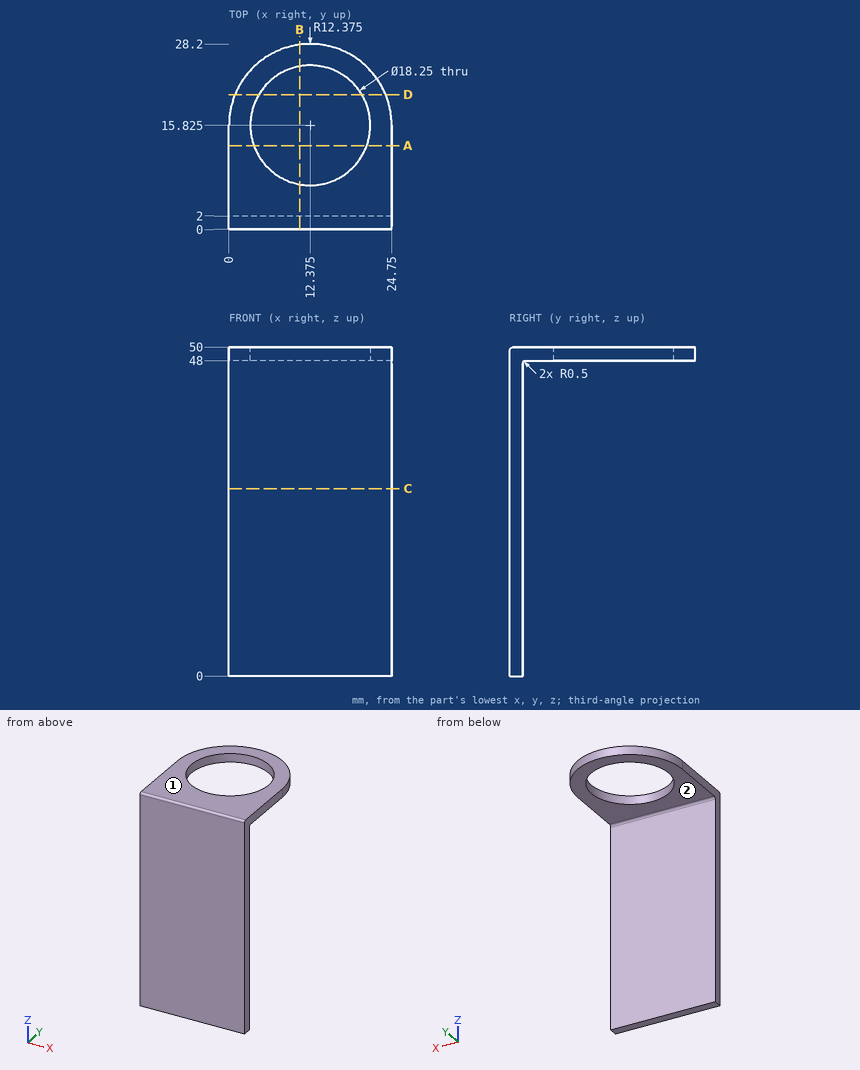
Input: dimensioned drawing with shaded views. Units: mm. Origin: part minimum x, y, z. A direction names the side the tool comes from. Round coordinates to 2 decimals unless told otherwise and drop trailing zeros. Loops run counter-clockwise (first coordinate to the right, second up) from the corner with the lowest first, then second, coordinate; pieces in that order, holes last. Notation, with made-up numbers: (36, -21.5) -> (88, -21.5) arc R17 cw to (88, -15.5) -> close; hole circle Ø3 at (-16, 8). An arc over 180 degrees is marked (long way). Answer as a JSON object with one key per item and string values. Group by question number.
1) Section query C-C on z = 28.5. Output: boundary loops of the cut face in (x, y).
2) Pin query (flat end, axial travel): pin 1 (10 mm diameter, centred on x = 21.5, z = 17.5, fed in from +Y); pin 2 (1.5 mm diameter, centred on x = 21.5, y = 8.5, fed in from -Z); pin 3 (1.5 mm diameter, centred on x = 5.5, y = 15.5, fed in from -Z) (1 decimal). Return the tip coordinate at first contact, or that it passes through.
3) Section query D-D on y = 20.5. Output: boundary loops of the cut face in (x, z), plus the area to 3 significant figures.
4) Ray query, L1, parallel to Z at x = 6, y = 4.5; L2, parallel to Y at x = 6, z = 44. Return the intervals inside material, ascending.
5) Reachability of the marked faces 1 and 2 from +Z, -Z, +X, -X, +Y, -Y: full face, straight path, thin tool, end or side. Return the list, or none.
6) Section query A-A on y = 12.75. Output: boundary loops of the cut face in (x, z), plus the area to 3 significant figures.
7) Section query B-B on x = 10.75. Output: boundary loops of the cut face in (y, z).
Reply:
{
 "1": {"outline": "(0, 0) -> (24.75, 0) -> (24.75, 2) -> (0, 2) -> close"},
 "2": {"pin 1": "stops at y = 2", "pin 2": "stops at z = 48", "pin 3": "passes through"},
 "3": {"outline": "(0.92, 48) -> (4.54, 48) -> (4.54, 50) -> (0.92, 50) -> close; (20.21, 48) -> (23.83, 48) -> (23.83, 50) -> (20.21, 50) -> close", "area": "14.5 mm2"},
 "4": {"L1": "z = 48 to 50", "L2": "y = 0 to 2"},
 "5": {"face 1": "+Z, +X, -X, +Y, -Y", "face 2": "-Z, +X, -X, +Y"},
 "6": {"outline": "(0, 48) -> (3.78, 48) -> (3.78, 50) -> (0, 50) -> close; (20.97, 48) -> (24.75, 48) -> (24.75, 50) -> (20.97, 50) -> close", "area": "15.1 mm2"},
 "7": {"outline": "(0, 0) -> (2, 0) -> (2, 47.5) arc R0.5 cw to (2.5, 48) -> (6.85, 48) -> (6.85, 50) -> (0.5, 50) arc R0.5 ccw to (0, 49.5) -> close; (24.8, 48) -> (28.09, 48) -> (28.09, 50) -> (24.8, 50) -> close"}
}
